Geometry check sheet. Reference: the model listing, model coordinates, mm. Round coordinates to 2 decimals unless told otherwise and drop trailing zeros. Write each loop counter-clockwise with the first axis right and the second up, starting at its lowest first coordinate (ties: lowest second). Pieces come first, ordered by that corner, then holes. Notation, with made-up numbers: M 68.25,22 L 77.25,22 A19 ccw 77.25,46 Z; hole C 70.25,-32 d10. An arc over 180 degrees is marked long. Put each result on its own line as item: value. Start each with the question number.
(1) Section check C-C on x = 4. Record the cut outline in (y, z).
(2) Section check A-A on z = 11. Record the cut outline in (x, y), then the cut area to 3 significant figures.
(3) Section check B-B on y = -7.5. Count the separate pieces of the cut face and the enclosed holes in it, then the cut area to 3 significant figures.
(4) Section check D-D on x = 48.5. Record the cut outline in (y, z).
(5) Material ranges on probe 1 along X at (y, z) = (-16, 46); probe 2 along X at (y, z) = (-7.75, 55); probe 3 along X at (y, z) = (-14, 3.5), recorded low to high.
(6) Gauge pin test, flat ends, axial feed: pin 1 (3 mm diameter, centred on x = 22.5, y = -16, fed in from -Z); pin 2 (3 mm diameter, centred on x = -44.5, y = -12, fed in from -Z); pin 3 (5 mm diameter, centred on x = 50.5, y = -14.5, fed in from -Z). Record the tip position at first contact, or that the pin passes through.
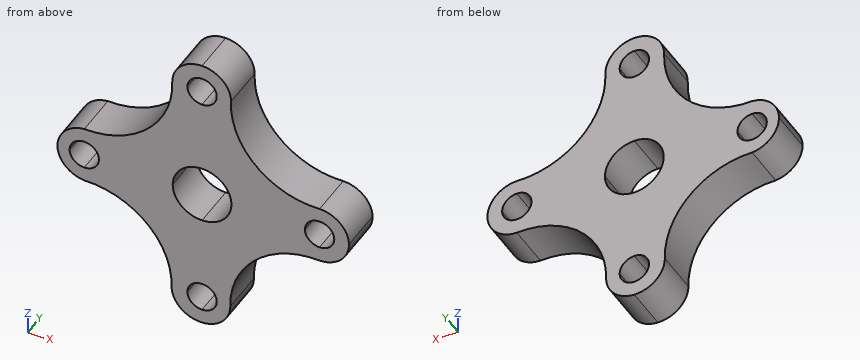
from build123d import *

# Parameters (mm, degrees)
F1_DEPTH = 19.05


with BuildPart() as f1:
    # F0 (on Front) → F1 (new body)
    with BuildSketch(Plane.XZ):
        with BuildLine():
            Line((44.433185, 0), (12.7, 0))
            ThreePointArc((12.7, 0), (8.980256, -8.980256), (0, -12.7))
            Line((0, -12.7), (0, -43.964499))
            ThreePointArc((0, -43.964499), (4.490128, -45.824371), (6.35, -50.314499))
            Line((6.35, -50.314499), (12.214499, -50.314499))
            ThreePointArc((12.214499, -50.314499), (23.286426, -23.137993), (50.783185, -12.887225))
            Line((50.783185, -12.887225), (50.783185, -6.35))
            ThreePointArc((50.783185, -6.35), (46.293057, -4.490128), (44.433185, 0))
        make_face()
        with BuildLine():
            ThreePointArc((0, 12.7), (8.980256, 8.980256), (12.7, 0))
            Line((12.7, 0), (44.433185, 0))
            ThreePointArc((44.433185, 0), (46.293057, 4.490128), (50.783185, 6.35))
            Line((50.783185, 6.35), (50.783185, 12.512775))
            ThreePointArc((50.783185, 12.512775), (23.230066, 23.111098), (12.520352, 50.621112))
            Line((12.520352, 50.621112), (6.35, 50.621112))
            ThreePointArc((6.35, 50.621112), (4.490128, 46.130984), (0, 44.271112))
            Line((0, 44.271112), (0, 12.7))
        make_face()
        with BuildLine():
            ThreePointArc((-12.7, 0), (-8.980256, 8.980256), (0, 12.7))
            Line((0, 12.7), (0, 44.271112))
            ThreePointArc((0, 44.271112), (-4.490128, 46.130984), (-6.35, 50.621112))
            Line((-6.35, 50.621112), (-12.879648, 50.621112))
            ThreePointArc((-12.879648, 50.621112), (-23.542161, 23.261338), (-50.902573, 12.600462))
            Line((-50.902573, 12.600462), (-50.902573, 6.35))
            ThreePointArc((-50.902573, 6.35), (-46.412445, 4.490128), (-44.552573, 0))
            Line((-44.552573, 0), (-12.7, 0))
        make_face()
        with BuildLine():
            Line((0, -43.964499), (0, -12.7))
            ThreePointArc((0, -12.7), (-8.980256, -8.980256), (-12.7, 0))
            Line((-12.7, 0), (-44.552573, 0))
            ThreePointArc((-44.552573, 0), (-46.412445, -4.490128), (-50.902573, -6.35))
            Line((-50.902573, -6.35), (-50.902573, -12.70329))
            ThreePointArc((-50.902573, -12.70329), (-23.898918, -23.34085), (-13.185501, -50.314499))
            Line((-13.185501, -50.314499), (-6.35, -50.314499))
            ThreePointArc((-6.35, -50.314499), (-4.490128, -45.824371), (0, -43.964499))
        make_face()
        with BuildLine():
            Line((50.783185, 12.512775), (50.783185, 6.35))
            ThreePointArc((50.783185, 6.35), (55.273313, 4.490128), (57.133185, 0))
            Line((57.133185, 0), (63.481805, 0))
            ThreePointArc((63.481805, 0), (59.697001, 8.858983), (50.783185, 12.512775))
        make_face()
        with BuildLine():
            ThreePointArc((57.133185, 0), (55.273313, -4.490128), (50.783185, -6.35))
            Line((50.783185, -6.35), (50.783185, -12.887225))
            ThreePointArc((50.783185, -12.887225), (59.829393, -9.101041), (63.481805, 0))
            Line((63.481805, 0), (57.133185, 0))
        make_face()
        with BuildLine():
            Line((-12.879648, 50.621112), (-6.35, 50.621112))
            ThreePointArc((-6.35, 50.621112), (-4.490128, 55.11124), (0, 56.971112))
            Line((0, 56.971112), (0, 63.319841))
            ThreePointArc((0, 63.319841), (-9.096163, 59.66466), (-12.879648, 50.621112))
        make_face()
        with BuildLine():
            ThreePointArc((0, 56.971112), (4.490128, 55.11124), (6.35, 50.621112))
            Line((6.35, 50.621112), (12.520352, 50.621112))
            ThreePointArc((12.520352, 50.621112), (8.8639, 59.537626), (0, 63.319841))
            Line((0, 63.319841), (0, 56.971112))
        make_face()
        with BuildLine():
            Line((12.214499, -50.314499), (6.35, -50.314499))
            ThreePointArc((6.35, -50.314499), (4.490128, -54.804627), (0, -56.664499))
            Line((0, -56.664499), (0, -63.005216))
            ThreePointArc((0, -63.005216), (8.664796, -59.121432), (12.214499, -50.314499))
        make_face()
        with BuildLine():
            ThreePointArc((0, -56.664499), (-4.490128, -54.804627), (-6.35, -50.314499))
            Line((-6.35, -50.314499), (-13.185501, -50.314499))
            ThreePointArc((-13.185501, -50.314499), (-9.292434, -59.464796), (0, -63.005216))
            Line((0, -63.005216), (0, -56.664499))
        make_face()
        with BuildLine():
            ThreePointArc((-57.252573, 0), (-55.392701, 4.490128), (-50.902573, 6.35))
            Line((-50.902573, 6.35), (-50.902573, 12.600462))
            ThreePointArc((-50.902573, 12.600462), (-59.143267, 8.548377), (-62.497918, 0))
            Line((-62.497918, 0), (-57.252573, 0))
        make_face()
        with BuildLine():
            Line((-50.902573, -12.70329), (-50.902573, -6.35))
            ThreePointArc((-50.902573, -6.35), (-55.392701, -4.490128), (-57.252573, 0))
            Line((-57.252573, 0), (-62.497918, 0))
            ThreePointArc((-62.497918, 0), (-59.178005, -8.613301), (-50.902573, -12.70329))
        make_face()
    extrude(amount=F1_DEPTH)


solid = f1.part
Answers follow:
1. outline: M -19.05,-62.2 L 0,-62.2 L 0,-55.25 L -19.05,-55.25 Z; M -19.05,-45.38 L 0,-45.38 L 0,-12.05 L -19.05,-12.05 Z; M -19.05,12.05 L 0,12.05 L 0,45.69 L -19.05,45.69 Z; M -19.05,55.55 L 0,55.55 L 0,62.61 L -19.05,62.61 Z
2. outline: M -56.06,-19.05 L -6.35,-19.05 L -6.35,0 L -56.06,0 Z; M 6.35,-19.05 L 56.79,-19.05 L 56.79,0 L 6.35,0 Z
2. area: 1,910 mm^2
3. separate pieces: 1
3. enclosed holes: 5
3. area: 5,600 mm^2
4. outline: M -19.05,-12.83 L 0,-12.83 L 0,-5.93 L -19.05,-5.93 Z; M -19.05,5.93 L 0,5.93 L 0,12.47 L -19.05,12.47 Z
5. probe 1: x = -12.98 to -4.36, 4.36 to 12.61
5. probe 2: x = -12.1 to -4.6, 4.6 to 11.74
5. probe 3: x = -61.99 to -56.2, -45.6 to -12.21, 12.21 to 45.48, 56.08 to 62.94
6. pin 1: stops at z = -25.57
6. pin 2: stops at z = -13.3
6. pin 3: stops at z = -12.89
